Geometry: final body of the model. Coordinates: model frame, mm. A direction names the side the tool comes from. Round coordinates to 2 decimals unless told otherwise and drop trailing zeros. Loops run counter-clockwise (first coordinate to the right, second up) from the corner with the lowest first, then second, coordinate; pieces in that order, holes last. Notation, with made-up numbers: (61, -28) -> (116, -28) arc R25 cw to (116, 3) -> close; hole circle Ø1 at (15, -23). An arc over 180 degrees is marked (long way). Answer in a Markdown table with one row per item.
Autodesk Inventor part; units mm, degrees
ref_plane "YZ Plane" through (0, 0, 0) normal (1, 0, 0) x (0, 1, 0)
ref_plane "XZ Plane" through (0, 0, 0) normal (0, 1, 0) x (-1, 0, 0)
ref_plane "XY Plane" through (0, 0, 0) normal (0, 0, 1) x (1, 0, 0)
sketch "Sketch1" plane through (0, 0, 0) normal (0, 0, 1) x (1, 0, 0)
  line L0 (0, 2.5) -> (0, 35)
  line L1 (0, 35) -> (50, 35)
  line L2 (50, 35) -> (50, 34)
  line L3 (50, 34) -> (60, 34)
  line L4 (60, 34) -> (60, 35)
  line L5 (60, 35) -> (110, 35)
  line L6 (110, 35) -> (110, 0)
  line L7 (110, 0) -> (30, 0)
  line L8 (0, 2.5) -> (30, 2.5)
  line L9 (30, 2.5) -> (30, 0)
  point P0 (0, 0)
  dimension "d1" = 1
  dimension "d2" = 10
  dimension "d3" = 50
  dimension "d4" = 50
  dimension "d5" = 1
  dimension "d8" = 2.5
  dimension "d9" = 35
  dimension "d10" = 30
  dimension "d12" = 30
  dimension "d14" = 110
revolve "Revolution1" add sketch "Sketch1" angle 360 about axis through (110, 0, 0) along (-1, 0, 0)
properties part number "CAM_demo" material "Aluminum 6061"
Item 1: Mould query, pull axis Z, two halves, no side actions, for faces 1 (the cylindrical face through (15.21, -0.54, -2.44)), 2 (the flat face through (30, 0, 0)), 3 (the cylindrical face through (85, -28, -21)), 4 (the flat face through (60, -5, -34)). Classes: released by +Z, released by -Z, zero draft, split by the parting line, or undercut.
Ans:
| item | result |
|---|---|
| face 1 | undercut |
| face 2 | undercut |
| face 3 | split by the parting line |
| face 4 | zero draft |
Item 2: First-contact query: P1, Ø10, axis at x = 27, y = 16.5, coming from the +Z side; P2, Ø4, axis at x = 58.5, y = -24.5, coming from the +Z side; P3, Ø10, axis at x = 22, z = 5.5, coming from the +Y side. Flat tips, straight axial feed; report the tip coordinate or a pass-through.
Ans:
| item | result |
|---|---|
| P1 | z = 33.06 |
| P2 | z = 26.23 |
| P3 | y = 35 |
Item 3: Section query D-D, the plane z = -13. Output: boundary loops of the cut face in (x, y).
Ans:
| item | result |
|---|---|
| outline | (0, -32.5) -> (50, -32.5) -> (50, -31.42) -> (60, -31.42) -> (60, -32.5) -> (110, -32.5) -> (110, 32.5) -> (60, 32.5) -> (60, 31.42) -> (50, 31.42) -> (50, 32.5) -> (0, 32.5) -> close |
Item 4: Ray query, L1, parallel to Z at x = 9, y = 0; L2, parallel to Y at x = 33, z = -6.5. Return the intervals inside material, ascending.
Ans:
| item | result |
|---|---|
| L1 | -35 to -2.5, 2.5 to 35 |
| L2 | -34.39 to 34.39 |
Item 5: Section query C-C, the plane x = 93. Output: boundary loops of the cut face in (y, z).
Ans:
| item | result |
|---|---|
| outline | circle Ø70 at (0, 0) |
Item 6: Set-up query: faces 5 (the flat face through (0, 0, 7)), 6 (the cylindrical face through (55.07, 18.28, 28.67)). Return all of +Z, -Z, +X, -X, +Y, -Y with unobstructed straight access to the full face (end or side cutting, diameter ignored); none if empty.
Ans:
| item | result |
|---|---|
| face 5 | +Z, -Z, -X, +Y, -Y |
| face 6 | none |
Item 7: Section query A-A, the plane z = 0. Output: boundary loops of the cut face in (x, y), and give its area (3 significant figures).
Ans:
| item | result |
|---|---|
| outline | (0, -35) -> (50, -35) -> (50, -34) -> (60, -34) -> (60, -35) -> (110, -35) -> (110, 35) -> (60, 35) -> (60, 34) -> (50, 34) -> (50, 35) -> (0, 35) -> (0, 2.5) -> (30, 2.5) -> (30, -2.5) -> (0, -2.5) -> close |
| area | 7,530 mm2 |
